The listing builds one solid part. Answer for the finished solid, in the listing's coordinates (mm). A direction names the side the tool comes from. Give positions to 0.01 mm unless a question says otherwise; leave off trailing zeros. Order: outer loops, then holes, each group sorted by start corner. A loop starts at its lowest first (then second) coordinate and runs counter-clockwise, first axis right, second up. Notation, with made-up numbers: (71, 24) - (126, 24) arc R20 cw to (126, 50) - close; hole circle Ø4 at (-10.75, 6). An arc over 180 degrees is marked (long way). Answer as a JSON object with one key per item and string values. Group by question number.
Q1. The mould has two halves that part along X. Classify faces 1 (the face through (-42, 2, 0)), 2 (the face through (46, 2, 0)), 3 (the face through (4, 3.5, 0)), 4 (the face through (-1, 0, 0)): released by +X, released by -X, zero draft, split by the parting line, or undercut.
Q2. A cutting plane is placed at D-D, the plane z = -15.5. Give the vertices of the cut face in (x, y), and give its area (3 significant figures).
Q3. A cutting plane is placed at C-C, the plane y = 2.55. Give the vertices of the cut face in (x, z).
Q4. Given pin 1 (7.5 mm diameter, centred on x = 14, z = 2, fed in from +Y); pin 2 (1.5 mm diameter, centred on x = -11, y = 2.5, fed in from +Z); pin 3 (1.5 mm diameter, centred on y = 3, z = -3, fed in from -X), each flat-ended and moving along its own axis, determine where each tip first touches the part or whether it passes through.
Q5. For faces 5 (the face through (1, 2, 10.5)), 6 (the face through (-5, 4, -9)), 7 (the face through (1, 2, -10.5)), determine the directions among +Z, -Z, +X, -X, +Y, -Y from which every point of the face is accessible in a straight line to the end or side of a thin tool.
Q6. Consider line 1 (X direction, y = 3.65, z = -6.5); line 2 (Z direction, x = 16, y = 3.6); line 3 (Z direction, x = 25, y = 1.35). Determine where each line is inside the solid, lowest interval first.
Q7. A cutting plane is placed at B-B, the plane z = 2. Give the vertices of the cut face in (x, y), and give its area (3 significant figures).
Q8. A cutting plane is placed at A-A, the plane x = -26.5. Give the vertices of the cut face in (y, z), and give its area (3 significant figures).
from build123d import *

# Parameters (mm, degrees)
SKETCH1_W           = 116
SKETCH1_H           = 37
BOSS_EXTRUDE1_DEPTH = 1
SKETCH2_W           = 88
SKETCH2_H           = 21
BOSS_EXTRUDE2_DEPTH = 3
SKETCH3_W           = 75.5
SKETCH3_H           = 14.6
CUT_EXTRUDE1_DEPTH  = 0.5


with BuildPart() as part:
    # Sketch1 → Boss-Extrude1 (new body)
    with BuildSketch(Plane(origin=(0, 0, 0), x_dir=(1, 0, 0), z_dir=(0, 1, 0))):
        Rectangle(SKETCH1_W, SKETCH1_H)
    extrude(amount=BOSS_EXTRUDE1_DEPTH)

    # Sketch2 → Boss-Extrude2 (add)
    with BuildSketch(Plane(origin=(0, 1, 0), x_dir=(1, 0, 0), z_dir=(0, 1, 0))):
        with Locations((2, 0)):
            Rectangle(SKETCH2_W, SKETCH2_H)
    extrude(amount=BOSS_EXTRUDE2_DEPTH)

    # Sketch3 → Cut-Extrude1 (cut)
    with BuildSketch(Plane(origin=(0, 4, 0), x_dir=(1, 0, 0), z_dir=(0, 1, 0))):
        with Locations((4.75, 0)):
            Rectangle(SKETCH3_W, SKETCH3_H)
    extrude(amount=-CUT_EXTRUDE1_DEPTH, mode=Mode.SUBTRACT)


solid = part.part
Reply:
{
 "1": {"face 1": "released by -X", "face 2": "released by +X", "face 3": "undercut", "face 4": "zero draft"},
 "2": {"outline": "(-58, 0) - (58, 0) - (58, 1) - (-58, 1) - close", "area": "116 mm^2"},
 "3": {"outline": "(-42, -10.5) - (46, -10.5) - (46, 10.5) - (-42, 10.5) - close"},
 "4": {"pin 1": "stops at y = 3.5", "pin 2": "stops at z = 10.5", "pin 3": "stops at x = -42"},
 "5": {"face 5": "+Z, +X, -X, +Y", "face 6": "+Z, -Z, +X, -X, +Y", "face 7": "-Z, +X, -X, +Y"},
 "6": {"line 1": "x = -42 to -33, 42.5 to 46", "line 2": "z = -10.5 to -7.3, 7.3 to 10.5", "line 3": "z = -10.5 to 10.5"},
 "7": {"outline": "(-58, 0) - (58, 0) - (58, 1) - (46, 1) - (46, 4) - (42.5, 4) - (42.5, 3.5) - (-33, 3.5) - (-33, 4) - (-42, 4) - (-42, 1) - (-58, 1) - close", "area": "342 mm^2"},
 "8": {"outline": "(0, -18.5) - (1, -18.5) - (1, -10.5) - (4, -10.5) - (4, -7.3) - (3.5, -7.3) - (3.5, 7.3) - (4, 7.3) - (4, 10.5) - (1, 10.5) - (1, 18.5) - (0, 18.5) - close", "area": "92.7 mm^2"}
}
